Verification items for the finished model (mm, model axes). A direction names the side the tool comes from. Round coordinates to 2 decimals unless told otherwise and drop trailing zeros. Loops run counter-clockwise (first coordinate to the right, second up) from the corner with the lowest first, then second, coordinate; pieces in that order, holes last. Notation, with made-up numbers: (84, -39.5) -> (105, -39.5) arc R24 cw to (105, -14.5) -> close; hole circle Ø11 at (77, 52.5). An arc over 180 degrees is marked (long way). Write item = value, one per line. Start each with the question number.
```python
from build123d import *

# Parameters (mm, degrees)
SKETCH1_W           = 40
SKETCH1_H           = 20
BOSS_EXTRUDE1_DEPTH = 1.75
SKETCH2_R           = 10
BOSS_EXTRUDE2_DEPTH = 18.8
SKETCH3_R           = 8.998930974
SKETCH3_R_2         = 3.75
CUT_EXTRUDE2_DEPTH  = 0.5
SKETCH4_R           = 1.519525434
CUT_EXTRUDE3_DEPTH  = 29.119432782
SKETCH5_R           = 1.494488577
SKETCH5_R_2         = 1.544110057
CUT_EXTRUDE5_DEPTH  = 1.75
SKETCH7_R           = 1.482162374
SKETCH7_R_2         = 1.476093664
BOSS_EXTRUDE3_DEPTH = 1.75
SKETCH8_R           = 0.972887348
SKETCH8_R_2         = 0.978406894
CUT_EXTRUDE6_DEPTH  = 29.680002664


with BuildPart() as part:
    # Sketch1 → Boss-Extrude1 (new body)
    with BuildSketch(Plane(origin=(0, 0, 0), x_dir=(1, 0, 0), z_dir=(0, 1, 0))):
        Rectangle(SKETCH1_W, SKETCH1_H)
    extrude(amount=BOSS_EXTRUDE1_DEPTH)

    # Sketch2 → Boss-Extrude2 (add)
    with BuildSketch(Plane(origin=(0, 0, 0), x_dir=(1, 0, 0), z_dir=(0, 1, 0))):
        with Locations(Location((-10, 0, 0), (0, 0, 270))):
            Circle(SKETCH2_R)
    extrude(amount=BOSS_EXTRUDE2_DEPTH)

    # Sketch3 → Cut-Extrude2 (cut)
    with BuildSketch(Plane(origin=(0, 18.8, 0), x_dir=(1, 0, 0), z_dir=(0, 1, 0))):
        with Locations(Location((-10, 0, 0), (0, 0, 270))):
            Circle(SKETCH3_R)
        with Locations(Location((-10, 0, 0), (0, 0, 270))):
            Circle(SKETCH3_R_2, mode=Mode.SUBTRACT)
    extrude(amount=-CUT_EXTRUDE2_DEPTH, mode=Mode.SUBTRACT)

    # Sketch4 → Cut-Extrude3 (cut, through all)
    with BuildSketch(Plane(origin=(0, 1.75, 0), x_dir=(1, 0, 0), z_dir=(0, 1, 0))):
        with Locations((20, 0)):
            Circle(SKETCH4_R)
    extrude(amount=-CUT_EXTRUDE3_DEPTH, mode=Mode.SUBTRACT)

    # Sketch5 → Cut-Extrude5 (cut)
    with BuildSketch(Plane.XZ):
        with Locations((-10, 10)):
            Circle(SKETCH5_R)
        with Locations((-10, -10)):
            Circle(SKETCH5_R_2)
    extrude(amount=-CUT_EXTRUDE5_DEPTH, mode=Mode.SUBTRACT)

    # Sketch7 → Boss-Extrude3 (add)
    with BuildSketch(Plane(origin=(0, 1.75, 0), x_dir=(1, 0, 0), z_dir=(0, 1, 0))):
        with Locations((11.99395038, -10)):
            Circle(SKETCH7_R)
        with Locations((11.99395038, 10)):
            Circle(SKETCH7_R_2)
    extrude(amount=-BOSS_EXTRUDE3_DEPTH)

    # Sketch8 → Cut-Extrude6 (cut, through all)
    with BuildSketch(Plane(origin=(0, 1.75, 0), x_dir=(1, 0, 0), z_dir=(0, 1, 0))):
        with Locations(Location((11.99395038, 10, 0), (0, 0, 270))):
            Circle(SKETCH8_R)
        with Locations(Location((11.99395038, -10, 0), (0, 0, 270))):
            Circle(SKETCH8_R_2)
    extrude(amount=-CUT_EXTRUDE6_DEPTH, mode=Mode.SUBTRACT)


solid = part.part
```
(1) Section check D-D on z = -1. Enter the section's corners in (x, y), then the cut area to 3 significant figures.
(2) Draft check along X on faces 1 (the flat face through (20, 1, -6)), 2 (the flat face through (-14, 18.3, 0)), 3 (the flat face through (-16, 1, -10)). Enter one of: +X half, -X half, draft (parallel to the pull), parting line (faces both ways), or undercut.
(3) Depth check by flat-ended pin: pin 1 Ø1.4 at (x, y) = (-17.5, 0.5) entering from -Z; pin 2 Ø5 at (x, z) = (4.5, 2.5) entering from +Y; pin 3 Ø8 at (y, z) = (14.5, 1) entering from +X. Enter the tip coordinate at first touch or a pass-through.
(4) Scan lines: line 1 (Y direction, x = 14, z = 0.25); line 2 (Y direction, x = -6, z = 2.5); line 3 (Z direction, x = -11.5, y = 17.5). Record each from-to range of solid material in increasing order. Write a range as [from, to].
(5) Section check C-C on x = -10. Enter the section's corners in (y, z), then the cut area to 3 significant figures.
(6) Section check B-B on y = 12.25. Enter the section's corners in (x, z).
(7) Access from +Z, -Z, +X, -X, +Y, -Y to the whole of each face (thin tool, end or side, straight path). Record for faces 4 (the flat face through (-18, 1.75, 8)), 5 (the flat face through (-10, 1.75, 9)), 6 (the flat face through (-18, 1.75, -8)).
(8) Section check A-A on x = 11.5. Enter the section's corners in (y, z), then the cut area to 3 significant figures.
Computed values:
q1.outline = (-20, 0) -> (18.86, 0) -> (18.86, 1.75) -> (-0.05, 1.75) -> (-0.05, 18.8) -> (-1.06, 18.8) -> (-1.06, 18.3) -> (-6.39, 18.3) -> (-6.39, 18.8) -> (-13.61, 18.8) -> (-13.61, 18.3) -> (-18.94, 18.3) -> (-18.94, 18.8) -> (-19.95, 18.8) -> (-19.95, 1.75) -> (-20, 1.75) -> close
q1.area = 402 mm²
q2.face_1 = +X half
q2.face_2 = undercut
q2.face_3 = draft
q3.pin_1 = -10
q3.pin_2 = 1.75
q3.pin_3 = 0
q4.line_1 = [0, 1.75]
q4.line_2 = [0, 18.3]
q4.line_3 = [-9.89, 9.89]
q5.outline = (0, -8.46) -> (1.75, -8.46) -> (1.75, -10) -> (18.8, -10) -> (18.8, -9) -> (18.3, -9) -> (18.3, -3.75) -> (18.8, -3.75) -> (18.8, 3.75) -> (18.3, 3.75) -> (18.3, 9) -> (18.8, 9) -> (18.8, 10) -> (1.75, 10) -> (1.75, 8.51) -> (0, 8.51) -> close
q5.area = 365 mm²
q6.outline = circle Ø20 at (-10, 0)
q7.face_4 = +Z, -X, +Y
q7.face_5 = +Z, -Y
q7.face_6 = -Z, -X, +Y
q8.outline = (0, -11.39) -> (1.75, -11.39) -> (1.75, -10.84) -> (0, -10.84) -> close; (0, -9.16) -> (1.75, -9.16) -> (1.75, 9.16) -> (0, 9.16) -> close; (0, 10.84) -> (1.75, 10.84) -> (1.75, 11.4) -> (0, 11.4) -> close
q8.area = 34.0 mm²
